from build123d import *

# Parameters (mm, degrees)
SKETCH1_W                      = 38.1
SKETCH1_H                      = 11.811
BOSS_EXTRUDE1_DEPTH            = 10.795
SKETCH2_W                      = 38.1
SKETCH2_H                      = 3.048
CUT_EXTRUDE1_DEPTH             = 3.175
F_1_4_0_25_PRESS_DOWEL_HOLE1_D = 6.35
F_10_32_TAPPED_HOLE1_D         = 4.0386


with BuildPart() as part:
    # Sketch1 → Boss-Extrude1 (new body)
    with BuildSketch(Plane(origin=(0, 0, 0), x_dir=(1, 0, 0), z_dir=(0, 1, 0))):
        with Locations((19.05, 5.9055)):
            Rectangle(SKETCH1_W, SKETCH1_H)
    extrude(amount=BOSS_EXTRUDE1_DEPTH)

    # Sketch2 → Cut-Extrude1 (cut)
    with BuildSketch(Plane(origin=(0, 10.795, 0), x_dir=(1, 0, 0), z_dir=(0, 1, 0))):
        with Locations((19.05, 10.287)):
            Rectangle(SKETCH2_W, SKETCH2_H)
    extrude(amount=-CUT_EXTRUDE1_DEPTH, mode=Mode.SUBTRACT)

    # 1/4 (0.25) Press Dowel Hole1 (through all)
    with Locations(Plane(origin=(0, 10.795, 0), x_dir=(1, 0, 0), z_dir=(0, 1, 0))):
        with Locations((7.62, 4.445), (30.48, 4.445)):
            Hole(F_1_4_0_25_PRESS_DOWEL_HOLE1_D / 2)

    # #10-32 Tapped Hole1 (through all)
    with Locations(Plane(origin=(0, 10.795, 0), x_dir=(1, 0, 0), z_dir=(0, 1, 0))):
        with Locations((19.05, 4.445)):
            Hole(F_10_32_TAPPED_HOLE1_D / 2)


solid = part.part
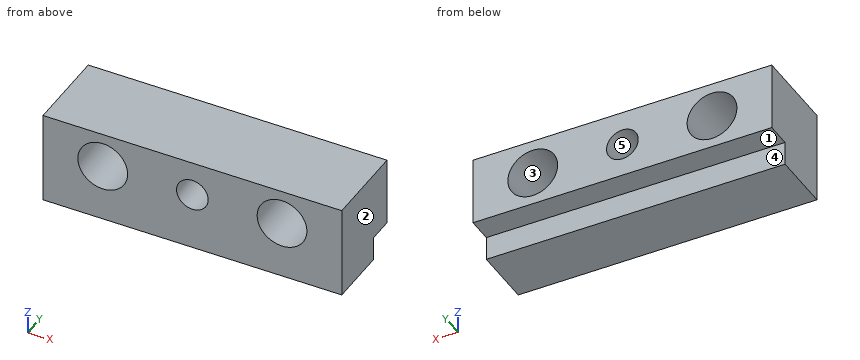
The listing builds one solid part. Answer for the finished solid, in the listing's coordinates (mm). Face numbers are marked on the shaded views. A direction names the side the tool comes from. Give positions to 0.01 mm unless a question says otherwise; leave off trailing zeros. Write each loop counter-clockwise with the first axis right and the second up, starting at its lowest first coordinate (ties: lowest second). Pieces come first, ordered by that corner, then holes. Notation, with made-up numbers: (34, 0) -> (54, 0) arc R25 cw to (54, 30) -> close; hole circle Ø8 at (-35, 62.25). An arc over 180 degrees is marked (long way). Use a Markdown table: item, result.
(1) Determine the mould class of the marked faces 1, 2 and 3 for opening direction X: released by +X, released by -X, zero draft, split by the parting line, or undercut.
Return value:
| item | result |
|---|---|
| face 1 | zero draft |
| face 2 | released by +X |
| face 3 | undercut |
(2) For the marked faces 4 and 5, determine the directions among +Z, -Z, +X, -X, +Y, -Y from which every point of the face is accessible in a straight line to the end or side of a thin tool.
Return value:
| item | result |
|---|---|
| face 4 | -Z, +X, -X, +Y |
| face 5 | +Y, -Y |
(3) Flat-ended cylindrical pins translate along their axes: P1, Ø3.5, axis at x = 18.5, z = -10, coming from the +Y side (3 decimals); P2, Ø1, axis at x = 16, y = 9, coming from the -Z side. Find the tip coordinate at first contact, or state that the pin passes through.
Return value:
| item | result |
|---|---|
| P1 | y = 10.795 |
| P2 | z = -8.76 |
(4) Find the intervals of material crossed by probe 1 along X at (y, z) = (8.5, -4.5); probe 2 along X at (y, z) = (8.5, -2.75); probe 3 along Z at (x, y) = (19.05, 4), in increasing order. Write a range as from..to.
Return value:
| item | result |
|---|---|
| probe 1 | 0..4.45, 10.79..17.03, 21.07..27.31, 33.65..38.1 |
| probe 2 | 0..4.94, 10.3..17.95, 20.15..27.8, 33.16..38.1 |
| probe 3 | -11.81..-6.46, -2.43..0 |
(5) Section D-D, the plane x = 35 is taken. Determine the outline of the cut face in (y, z) (3 decimals), then the cut area to 3 significant figures.
Return value:
| item | result |
|---|---|
| outline | (0, -11.811) -> (7.62, -11.811) -> (7.62, -8.763) -> (10.795, -8.763) -> (10.795, 0) -> (0, 0) -> close |
| area | 118 mm2 |
(6) Section C-C, the plane y = 1.25 is taken. Determine the outline of the cut face in (x, z) (3 decimals).
Return value:
| item | result |
|---|---|
| outline | (0, -11.811) -> (38.1, -11.811) -> (38.1, 0) -> (0, 0) -> close; hole circle Ø6.35 at (7.62, -4.445); hole circle Ø4.039 at (19.05, -4.445); hole circle Ø6.35 at (30.48, -4.445) |
(7) Section A-A, the plane x = 19.05 is taken. Determine the outline of the cut face in (y, z) (3 decimals).
Return value:
| item | result |
|---|---|
| outline | (0, -11.811) -> (7.62, -11.811) -> (7.62, -8.763) -> (10.795, -8.763) -> (10.795, -6.464) -> (0, -6.464) -> close; (0, -2.426) -> (10.795, -2.426) -> (10.795, 0) -> (0, 0) -> close |
(8) Section B-B, the plane z = -7 is taken. Determine the outline of the cut face in (x, y) (3 decimals), then the cut area to 3 significant figures.
Return value:
| item | result |
|---|---|
| outline | (0, 0) -> (5.735, 0) -> (5.735, 10.795) -> (0, 10.795) -> close; (9.505, 0) -> (28.595, 0) -> (28.595, 10.795) -> (9.505, 10.795) -> close; (32.365, 0) -> (38.1, 0) -> (38.1, 10.795) -> (32.365, 10.795) -> close |
| area | 330 mm2 |
